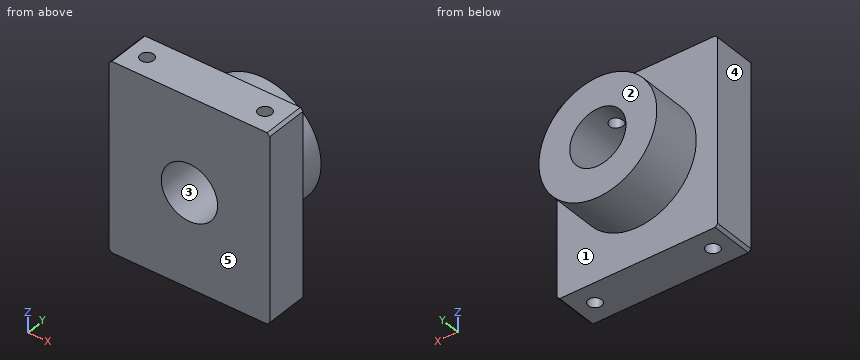
from build123d import *

# Parameters (mm, degrees)
SKETCH_1_W                  = 30
SKETCH_1_H                  = 35
EXTRUDE_1_DEPTH             = 10
SKETCH_3_R                  = 11
SKETCH_3_R_2                = 5.25
EXTRUDE_2_DEPTH             = 8.5
CHAMFER_1_SIZE              = 0.5
SKETCH_6_R                  = 5.25
CUT_EXTRUDE_3_DEPTH         = 30.555033412
SKETCH_7_W                  = 31.194113832
SKETCH_7_H                  = 36.870983812
CUT_EXTRUDE_4_DEPTH         = 1
CUT_EXTRUDE_START           = -1
SKETCH_8_W                  = 33.487798672
SKETCH_8_H                  = 37.788457748
SKETCH_8_R                  = 11
CUT_EXTRUDE_5_DEPTH         = 1
HOLE_WIZARD_M3_1_AT_2_COUNT = 2
HOLE_WIZARD_M3_1_AT_2_PITCH = 22
SKETCH_4_R                  = 1.25
CUT_EXTRUDE_6_DEPTH         = 30.555033412


with BuildPart() as part:
    # 草图1 → 凸台-拉伸1 (new body)
    with BuildSketch(Plane(origin=(0, 0, 0), x_dir=(1, 0, 0), z_dir=(0, 1, 0))):
        Rectangle(SKETCH_1_W, SKETCH_1_H)
    extrude(amount=EXTRUDE_1_DEPTH)

    # 草图3 → 凸台-拉伸2 (add)
    with BuildSketch(Plane(origin=(0, 10, 0), x_dir=(1, 0, 0), z_dir=(0, 1, 0))):
        with Locations(Location((0, 0, 0), (0, 0, 270))):
            Circle(SKETCH_3_R)
        with Locations(Location((0, 0, 0), (0, 0, 270))):
            Circle(SKETCH_3_R_2, mode=Mode.SUBTRACT)
    extrude(amount=EXTRUDE_2_DEPTH)

    # 倒角1
    chamfer_1_edges = [part.edges().sort_by_distance(p)[0] for p in [
        (15, 5, 17.5),
        (-15, 5, 17.5),
        (-15, 5, -17.5),
        (15, 5, -17.5),
    ]]
    chamfer(chamfer_1_edges, length=CHAMFER_1_SIZE)

    # 草图6 → 切除-拉伸3 (cut, through all)
    with BuildSketch(Plane(origin=(0, 18.5, 0), x_dir=(1, 0, 0), z_dir=(0, 1, 0))):
        with Locations(Location((0, 0, 0), (0, 0, 270))):
            Circle(SKETCH_6_R)
    extrude(amount=-CUT_EXTRUDE_3_DEPTH, mode=Mode.SUBTRACT)

    # 草图7 → 切除-拉伸4 (cut)
    with BuildSketch(Plane.XZ):
        Rectangle(SKETCH_7_W, SKETCH_7_H)
    extrude(amount=-CUT_EXTRUDE_4_DEPTH, mode=Mode.SUBTRACT)

    # 草图8 → 切除-拉伸5 (cut)
    with BuildSketch(Plane(origin=(0, 10, 0), x_dir=(1, 0, 0), z_dir=(0, 1, 0)).offset(CUT_EXTRUDE_START)):
        Rectangle(SKETCH_8_W, SKETCH_8_H)
        with Locations(Location((0, 0, 0), (0, 0, 270))):
            Circle(SKETCH_8_R, mode=Mode.SUBTRACT)
    extrude(amount=CUT_EXTRUDE_5_DEPTH, mode=Mode.SUBTRACT)

    # 草图9 → M3 螺纹孔1 (revolve, cut)
    with BuildSketch(Plane(origin=(-11, 5, 17.5), x_dir=(0, -1, 0), z_dir=(1, 0, 0))):
        Polygon((0, 0), (0, 8.751075774), (1.25, 8), (1.25, 0), align=None)
    hole_wizard_m3_1 = revolve(axis=Axis((-11, 5, 23.85), (0, 0, -1)), mode=Mode.SUBTRACT)

    # M3 螺纹孔1 at 2: M3 螺纹孔1 ×2
    with Locations(*[(i * HOLE_WIZARD_M3_1_AT_2_PITCH, 0, 0) for i in range(1, HOLE_WIZARD_M3_1_AT_2_COUNT)]):
        add(hole_wizard_m3_1, mode=Mode.SUBTRACT)

    # 镜向1: M3 螺纹孔1 across plane
    add(hole_wizard_m3_1.mirror(Plane.XY), mode=Mode.SUBTRACT)

    # 镜向1 copy 1 sketch → 镜向1 copy 1 (revolve, cut)
    with BuildSketch(Plane(origin=(11, 5, -17.5), x_dir=(0, -1, 0), z_dir=(1, 0, 0))):
        Polygon((0, 0), (0, -8.751075774), (1.25, -8), (1.25, 0), align=None)
    revolve(axis=Axis((11, 5, -23.85), (0, 0, -1)), mode=Mode.SUBTRACT)

    # 草图4 → 切除-拉伸6 (cut, through all)
    with BuildSketch(Plane.XY):
        with Locations(Location((0, 14, 0), (0, 0, 180))):
            Circle(SKETCH_4_R)
    extrude(amount=CUT_EXTRUDE_6_DEPTH, mode=Mode.SUBTRACT)


solid = part.part
Geometry check sheet. Reference: the model listing, model coordinates, mm. Face numbers are marked on the shaded views. A direction names the side the tool comes from. Give positions to 0.01 mm unless a question says otherwise; leave off trailing zeros. Order: outer loops, then holes, each group sorted by start corner. A loop starts at its lowest first (then second) coordinate and runs counter-clockwise, first axis right, second up.
1) Tool access check on the marked faces 1 and 2. Record the directions out of +Z, -Z, +X, -X, +Y, -Y that give a thin tool (end or side, any length) a straight path to the whole face; none if there is none.
Results are:
face 1: +Y
face 2: +Z, -Z, +X, -X, +Y
2) Gauge pin test, flat ends, axial feed: pin 1 (1.5 mm diameter, centred on x = -5, z = -11.5, fed in from +Y); pin 2 (1.5 mm diameter, centred on x = 11, y = 5, fed in from +Z); pin 3 (10 mm diameter, centred on x = 11, z = -7, fed in from +Y); pin 4 (3 mm diameter, centred on x = 0, y = 14, fed in from -Z). Record the tip position at first contact, or that the pin passes through.
Results are:
pin 1: stops at y = 9
pin 2: stops at z = 9.2
pin 3: stops at y = 18.5
pin 4: stops at z = -11
3) Cross-section at B-B (y = 7). Record the boundary of the cut face in (x, z), then the cut area to 3 significant figures.
Results are:
outline: (-15, -17) - (-14.5, -17.5) - (14.5, -17.5) - (15, -17) - (15, 17) - (14.5, 17.5) - (-14.5, 17.5) - (-15, 17) - close; hole circle Ø10.5 at (0, 0)
area: 963 mm2
4) Draft check along X on the marked faces 3, 4 and 5. Enter one of: released by +X, released by -X, zero draft, split by the parting line, or undercut.
Results are:
face 3: undercut
face 4: released by -X
face 5: zero draft
5) Material ranges on probe 1 along X at (y, z) = (5, -15.25); probe 2 along Z at (x, y) = (0.25, 7.5); probe 3 along Y at (x, z) = (-11, 12.5), recorded low to high.
Results are:
probe 1: x = -15 to -12.25, -9.75 to 9.75, 12.25 to 15
probe 2: z = -17.5 to -5.24, 5.24 to 17.5
probe 3: y = 1 to 3.75, 6.25 to 9
6) Cross-section at A-A (x = 0). Record the boundary of the cut face in (y, z).
Results are:
outline: (1, -17.5) - (9, -17.5) - (9, -11) - (18.5, -11) - (18.5, -5.25) - (1, -5.25) - close; (1, 5.25) - (12.75, 5.25) - (12.75, 11) - (9, 11) - (9, 17.5) - (1, 17.5) - close; (15.25, 5.25) - (18.5, 5.25) - (18.5, 11) - (15.25, 11) - close
7) Cross-section at C-C (z = 0). Record the boundary of the cut face in (x, y), then the cut area to 3 significant figures.
Results are:
outline: (-15, 1) - (-5.25, 1) - (-5.25, 18.5) - (-11, 18.5) - (-11, 9) - (-15, 9) - close; (5.25, 1) - (15, 1) - (15, 9) - (11, 9) - (11, 18.5) - (5.25, 18.5) - close
area: 265 mm2
8) Cross-section at D-D (z = 10). Record the boundary of the cut face in (x, y), then the cut area to 3 significant figures.
Results are:
outline: (-15, 1) - (15, 1) - (15, 9) - (4.58, 9) - (4.58, 18.5) - (-4.58, 18.5) - (-4.58, 9) - (-15, 9) - close; hole circle Ø2.5 at (-11, 5); hole circle Ø2.5 at (0, 14); hole circle Ø2.5 at (11, 5)
area: 312 mm2
